For this review, take the finished solid that the model builds, in its own axes (mm). Round coordinates to 2 decimals unless told otherwise and drop trailing zeros. Write each loop counter-clockwise with the first axis right and the second up, starting at its lowest first coordinate (ties: lowest second). Pieces come first, ordered by that corner, then holes.
from build123d import *

# Parameters (mm, degrees)
CUT_EXTRUDE_1_DEPTH = 6.662375826


with BuildPart() as part:
    # ｽｹｯﾁ1 → 回転1 (revolve)
    with BuildSketch(Plane.XY, mode=Mode.PRIVATE) as revolve_1_sk:
        Polygon((1.25, 0), (1.25, 2.75), (3, 2.75), (3, 1.15), (3.5, 1.15), (3.5, 0), align=None)
    revolve(revolve_1_sk.sketch.rotate(Axis((0, 0, 0), (0, 1, 0)), 90), axis=Axis((0, 0, 0), (0, 1, 0)))

    # ｽｹｯﾁ2 → ｶｯﾄ - 押し出し1 (cut, through all)
    with BuildSketch(Plane(origin=(0, 2.75, 0), x_dir=(1, 0, 0), z_dir=(0, 1, 0))):
        with BuildLine():
            Line((-2.939387691, -1.9), (2.939387691, -1.9))
            ThreePointArc((2.939387691, -1.9), (0, -3.5), (-2.939387691, -1.9))
        make_face()
    extrude(amount=-CUT_EXTRUDE_1_DEPTH, mode=Mode.SUBTRACT)


solid = part.part
(1) We need section D-D, the plane z = -2.9. Give the boundary of the cut face in (x, y), and give its area (3 significant figures).
Geometry check:
outline: (-1.96, 0) - (1.96, 0) - (1.96, 1.15) - (0.77, 1.15) - (0.77, 2.75) - (-0.77, 2.75) - (-0.77, 1.15) - (-1.96, 1.15) - close
area: 6.97 mm2
(2) We need section C-C, the plane x = 2.5. Give the boundary of the cut face in (y, z).
Geometry check:
outline: (0, -2.45) - (1.15, -2.45) - (1.15, -1.66) - (2.75, -1.66) - (2.75, 1.66) - (1.15, 1.66) - (1.15, 1.9) - (0, 1.9) - close
(3) Mouldability with a two-part tool opening along Z and no side actions: class faces 1 (the face through (-1, 1.15, -3)), 2 (the face through (0, 1, 1.9)), 3 (the face through (-0.05, 1.39, 1.25)), 4 (the face through (0, 2, -3)) as pulls with the +Z half, pulls with the -Z half, needs draft (parallel to the pull), parting line crosses it, or undercut.
Geometry check:
face 1: needs draft
face 2: pulls with the +Z half
face 3: undercut
face 4: parting line crosses it
(4) For line 1 along X through (y, z) = (1.75, 0); line 2 along X through (y, z) = (2.4, -0.75); line 3 along Z through (x, y) = (0.5, 1.3), list the stretches that pass through material, from the lowest coordinate up.
Geometry check:
line 1: x = -3 to -1.25, 1.25 to 3
line 2: x = -2.9 to -1, 1 to 2.9
line 3: z = -2.96 to -1.15, 1.15 to 1.9
(5) We need section A-A, the plane z = 0. Give the boundary of the cut face in (x, y), and give its area (3 significant figures).
Geometry check:
outline: (-3.5, 0) - (-1.25, 0) - (-1.25, 2.75) - (-3, 2.75) - (-3, 1.15) - (-3.5, 1.15) - close; (1.25, 0) - (3.5, 0) - (3.5, 1.15) - (3, 1.15) - (3, 2.75) - (1.25, 2.75) - close
area: 10.8 mm2
(6) We need section B-B, the plane x = 0. Give the boundary of the cut face in (y, z).
Geometry check:
outline: (0, -3.5) - (1.15, -3.5) - (1.15, -3) - (2.75, -3) - (2.75, -1.25) - (0, -1.25) - close; (0, 1.25) - (2.75, 1.25) - (2.75, 1.9) - (0, 1.9) - close
